Read the model definition and answer for the solid it produces. Units are mm, in the model's axes. Face numbers are marked on the shaded views. A direction names the side the tool comes from. Coordinates: 2 decimals unless noted, no trailing zeros. Write each loop counter-clockwise with the first axis right and the second up, starting at its lowest first coordinate (ties: lowest second). Pieces come first, ordered by that corner, then holes.
(1) Section D-D on z = 2.75 is taken. Write down the section's boundary in (x, y), then the cut area to 3 significant figures.
(2) Section A-A on z = 10 is taken. Write down the section's boundary in (x, y) (3 decimals).
(3) Given pin 1 (0.9 mm diameter, centred on x = 1.5, z = 10.5, fed in from +Y); pin 2 (0.6 mm diameter, centred on y = 0, z = 10, fed in from -X); pin 3 (2 mm diameter, centred on y = -2, z = 9.5, fed in from +X), each flat-ended and moving along its own axis, determine where each tip first touches the part or whether it passes through.
(4) Section C-C on x = -1.5 is taken. Write down the section's boundary in (y, z) (3 decimals).
(5) Section B-B on y = -3.25 is taken. Write down the section's boundary in (x, z), then the cut area to 4 significant figures.
(6) Find the intervals of material crossed by probe 1 along Y at (x, z) = (-1.75, 8) (3 decimals); probe 2 along Y at (x, z) = (1, 5); probe 3 along Z at (x, y) = (6, -4.5), in increasing order.
(7) Which of the six approach directions +Z, -Z, +X, -X, +Y, -Y give full straight-line access (tool end or side, diameter ignored) to the marked faces 1, 2, 3 and 4?
from build123d import *

# Parameters (mm, degrees)
PAD_DEPTH    = 3
SKETCH001_W  = 7
SKETCH001_H  = 5.5
PAD001_DEPTH = 9
POCKET_DEPTH = 5
CHAMFER_SIZE = 1


with BuildPart() as part:
    # Sketch → Pad (new body)
    with BuildSketch(Plane.XY):
        with BuildLine():
            ThreePointArc((-6.25, 8.75), (-8.017767, 8.017767), (-8.75, 6.25))
            Line((-8.75, -6.25), (-8.75, 6.25))
            ThreePointArc((-8.75, -6.25), (-8.017767, -8.017767), (-6.25, -8.75))
            Line((6.25, -8.75), (-6.25, -8.75))
            ThreePointArc((6.25, -8.75), (8.017767, -8.017767), (8.75, -6.25))
            Line((8.75, 6.25), (8.75, -6.25))
            ThreePointArc((8.75, 6.25), (8.017767, 8.017767), (6.25, 8.75))
            Line((-6.25, 8.75), (6.25, 8.75))
        make_face()
    extrude(amount=PAD_DEPTH)

    # Sketch001 (on Face10 of Pad) → Pad001 (join)
    with BuildSketch(Plane.XY.offset(3)):
        Rectangle(SKETCH001_W, SKETCH001_H)
    extrude(amount=PAD001_DEPTH)

    # Sketch002 (on Face15 of Pad001) → Pocket (cut)
    with BuildSketch(Plane.XY.offset(12)):
        with BuildLine():
            Line((-0.625, 2.75), (-0.625, 0.925))
            ThreePointArc((-0.925, 0.625), (-0.712868, 0.712868), (-0.625, 0.925))
            Line((-0.925, 0.625), (-2.1, 0.625))
            Line((-2.1, 0.625), (-2.1, -0.625))
            Line((-2.1, -0.625), (-0.925, -0.625))
            ThreePointArc((-0.625, -0.925), (-0.712868, -0.712868), (-0.925, -0.625))
            Line((-0.625, -0.925), (-0.625, -2.75))
            Line((-0.625, -2.75), (0.625, -2.75))
            Line((0.625, -0.925), (0.625, -2.75))
            ThreePointArc((0.925, -0.625), (0.712868, -0.712868), (0.625, -0.925))
            Line((2.1, -0.625), (0.925, -0.625))
            Line((2.1, 0.625), (2.1, -0.625))
            Line((0.925, 0.625), (2.1, 0.625))
            ThreePointArc((0.625, 0.925), (0.712868, 0.712868), (0.925, 0.625))
            Line((0.625, 2.75), (0.625, 0.925))
            Line((-0.625, 2.75), (0.625, 2.75))
        make_face()
    extrude(amount=-POCKET_DEPTH, mode=Mode.SUBTRACT)

    # Chamfer
    chamfer_edges = [part.edges().sort_by_distance(p)[0] for p in [
        (-3.5, 0, 3),
        (0, 2.75, 3),
        (0, -2.75, 3),
        (3.5, 0, 3),
    ]]
    chamfer(chamfer_edges, length=CHAMFER_SIZE)


solid = part.part
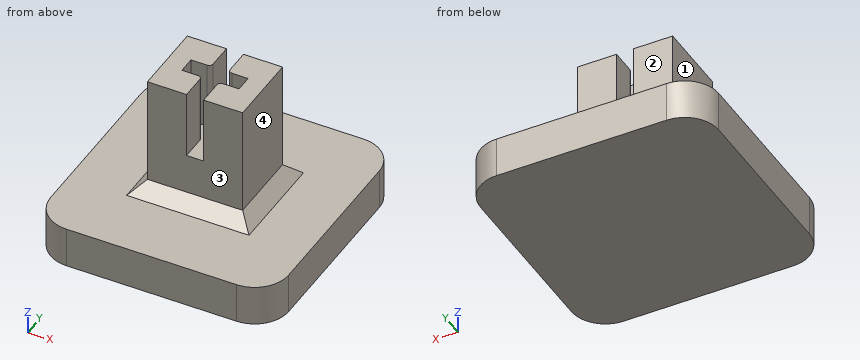
Response:
1. outline: (-8.75, -6.25) arc R2.5 ccw to (-6.25, -8.75) - (6.25, -8.75) arc R2.5 ccw to (8.75, -6.25) - (8.75, 6.25) arc R2.5 ccw to (6.25, 8.75) - (-6.25, 8.75) arc R2.5 ccw to (-8.75, 6.25) - close
1. area: 301 mm2
2. outline: (-3.5, -2.75) - (-0.625, -2.75) - (-0.625, -0.925) arc R0.3 ccw to (-0.925, -0.625) - (-2.1, -0.625) - (-2.1, 0.625) - (-0.925, 0.625) arc R0.3 ccw to (-0.625, 0.925) - (-0.625, 2.75) - (-3.5, 2.75) - close; (0.625, -2.75) - (3.5, -2.75) - (3.5, 2.75) - (0.625, 2.75) - (0.625, 0.925) arc R0.3 ccw to (0.925, 0.625) - (2.1, 0.625) - (2.1, -0.625) - (0.925, -0.625) arc R0.3 ccw to (0.625, -0.925) - close
3. pin 1: stops at y = 2.75
3. pin 2: stops at x = -3.5
3. pin 3: stops at x = 3.5
4. outline: (-8.75, 0) - (8.75, 0) - (8.75, 3) - (3.75, 3) - (2.75, 4) - (2.75, 12) - (0.625, 12) - (0.625, 7) - (-0.625, 7) - (-0.625, 12) - (-2.75, 12) - (-2.75, 4) - (-3.75, 3) - (-8.75, 3) - close
5. outline: (-8.75, 0) - (8.75, 0) - (8.75, 3) - (4.5, 3) - (4, 3.5) - (-4, 3.5) - (-4.5, 3) - (-8.75, 3) - close
5. area: 56.75 mm2
6. probe 1: y = -2.75 to -0.625, 0.625 to 2.75
6. probe 2: y = -2.75 to 2.75
6. probe 3: z = 0 to 3
7. face 1: +Z, -X, +Y, -Y
7. face 2: +Z, +X, -X, +Y
7. face 3: +Z, +X, -X, -Y
7. face 4: +Z, +X, +Y, -Y
